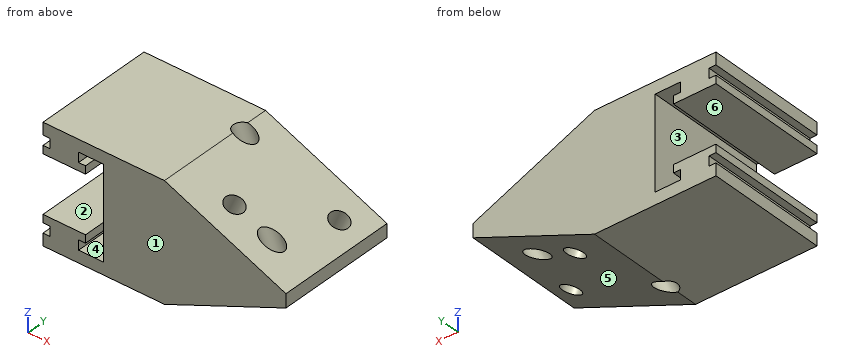
Autodesk Inventor part; units mm, degrees
ref_plane "YZ Plane" through (0, 0, 0) normal (1, 0, 0) x (0, 1, 0)
ref_plane "XZ Plane" through (0, 0, 0) normal (0, 1, 0) x (-1, 0, 0)
ref_plane "XY Plane" through (0, 0, 0) normal (0, 0, 1) x (1, 0, 0)
sketch "Sketch1" plane through (0, 0, 0) normal (0, 1, 0) x (-1, 0, 0)
  line L0 (0, 0) -> (-12.7, 0)
  line L1 (-12.7, 0) -> (-12.7, -2.54)
  line L2 (-12.7, -2.54) -> (0, -2.54)
  line L3 (0, -2.54) -> (0, 0)
  line L4 (0, -21.844) -> (-12.7, -21.844)
  line L5 (-12.7, -21.844) -> (-12.7, -24.384)
  line L6 (-12.7, -24.384) -> (0, -24.384)
  line L7 (0, -24.384) -> (0, -21.844)
  line L8 (-12.7, 0) -> (-25.4, 0)
  line L9 (-25.4, 0) -> (-25.4, -24.384)
  line L10 (-25.4, -24.384) -> (-12.7, -24.384)
  line L11 (-12.7, -24.384) -> (-12.7, 0)
  line L12 (-25.4, 0) -> (-50.8, -10.7817)
  line L13 (-25.4, 0) -> (2.1936, 0) construction
  line L14 (-25.4, -24.384) -> (-50.8, -13.6023)
  line L15 (-25.4, -24.384) -> (2.1936, -24.384) construction
  line L16 (-50.8, -10.7817) -> (-50.8, -13.6023)
  line L17 (-1.4478, -4.572) -> (-7.4422, -4.572)
  line L18 (-7.4422, -4.572) -> (-7.4422, -2.54)
  line L19 (-7.4422, -2.54) -> (-1.4478, -2.54)
  line L20 (-1.4478, -2.54) -> (-1.4478, -4.572)
  line L21 (-1.4478, -21.844) -> (-7.4422, -21.844)
  line L22 (-7.4422, -21.844) -> (-7.4422, -19.812)
  line L23 (-7.4422, -19.812) -> (-1.4478, -19.812)
  line L24 (-1.4478, -19.812) -> (-1.4478, -21.844)
  line L25 (0, -19.812) -> (-8.89, -19.812)
  line L26 (-8.89, -19.812) -> (-8.89, -18.161)
  line L27 (-8.89, -18.161) -> (0, -18.161)
  line L28 (0, -18.161) -> (0, -19.812)
  line L29 (0, -4.572) -> (-8.89, -4.572)
  line L30 (-8.89, -4.572) -> (-8.89, -6.223)
  line L31 (-8.89, -6.223) -> (0, -6.223)
  line L32 (0, -6.223) -> (0, -4.572)
  dimension "d2" = 12.7
  dimension "d3" = 2.54
  dimension "d4" = 12.7
  dimension "d5" = 2.54
  dimension "d6" = 24.384
  dimension "d7" = 12.7
  dimension "d8" = 24.384
  dimension "d9" = 157
  dimension "d10" = 157
  dimension "d11" = 25.4
  dimension "d12" = 25.4
  dimension "d15" = 5.9944
  dimension "d16" = 2.032
  dimension "d17" = 2.032
  dimension "d18" = 1.4478
  dimension "d19" = 5.9944
  dimension "d20" = 2.032
  dimension "d21" = 1.4478
  dimension "d22" = 8.89
  dimension "d23" = 1.651
  dimension "d24" = 8.89
  dimension "d25" = 1.651
extrude "Extrusion1" add sketch "Sketch1" along normal blind 25.4
sketch "Sketch2" plane through (25.4, 0, -24.384) normal (0.3907, 0, -0.9205) x (-0.9205, 0, -0.3907)
  circle A0 centre (-10.16, 19.05) radius 1.9685
  circle A1 centre (-22.5136, 6.35) radius 1.9685
  line L0 (-27.5936, 0) -> (0, 0)
  line L1 (-27.5936, 0) -> (-27.5936, 25.4)
  line L2 (0, 0) -> (0, 25.4)
  line L3 (-27.5936, 25.4) -> (0, 25.4)
  point P0 (13.8532, 0)
  dimension "d28" = 3.937
  dimension "d29" = 3.937
  dimension "d30" = 6.35
  dimension "d31" = 5.08
  dimension "d32" = 10.16
  dimension "d33" = 6.35
hole "Hole1" at (34.7523, 19.05, -20.4142) at (46.1238, 6.35, -15.5873) direction (-0.3907, 0, 0.9205) diameter 3.937 end through all
sketch "Sketch3" plane through (50.8, 0, -10.7817) normal (0.3907, 0, 0.9205) x (0.9205, 0, -0.3907)
  circle A0 centre (-5.08, 19.05) radius 1.9685
  circle A1 centre (-17.4336, 6.35) radius 1.9685
  line L0 (-27.5936, 25.4) -> (0, 25.4)
  line L1 (0, 0) -> (0, 25.4)
  line L2 (-27.5936, 0) -> (0, 0)
  line L3 (-27.5936, 0) -> (-27.5936, 17.1859)
  point P0 (-50.9744, 0)
  dimension "d41" = 3.937
  dimension "d42" = 3.937
  dimension "d43" = 6.35
  dimension "d44" = 5.08
  dimension "d45" = 6.35
  dimension "d46" = 10.16
hole "Hole2" at (46.1238, 19.05, -8.7967) at (34.7523, 6.35, -3.9698) direction (-0.3907, 0, -0.9205) diameter 3.937 end through all
ref_plane "Work Plane1" through (47.8226, 0, -17.7959) normal (0.3907, 0, 0.9205) x (0.9205, 0, -0.3907)
properties part number "XRailSplitter"
Check sheet for the modelled part. Datum: model origin and axes. Units: mm. Face numbers are marked on the shaded views. A direction names the side the tool comes from. Give positions to 0.01 mm unless a question says otherwise; leave off trailing zeros. Order: outer loops, then holes, each group sorted by start corner. A loop starts at its lowest first (then second) coordinate and runs counter-clockwise, first axis right, second up. Notation, with made-up numbers: M -23.75,79.25 L 33.25,79.25 A15 cw 33.25,95.25 Z; hole C -15,10.25 d8. An arc over 180 degrees is marked long. Answer in a Markdown table with one row per item. Add a question column.
Q1. Release check for a two-part mould opening along X. For the marked faces 3, 4, 5 and 6 record: released by +X, released by -X, zero draft, split by the parting line, or undercut.
Q2. Access from +Z, -Z, +X, -X, +Y, -Y to the whole of each face (thin tool, end or side, straight path). Record for the marked faces 1 and 2.
Q3. Thickness scan on L1, parallel to Z at x = 6, y = 22; L2, parallel to X at y = 18, z = -5.5; L3, parallel to Y at x = 28, z = -2.5. Record the ranges inside material, lowest first.
Q4. Sectioned sample at A-A, the plane y = 23.75. Record the boundary of the cut face in (x, z).
Q5. Gauge pin test, flat ends, axial feed: pin 1 Ø10 at (y, z) = (3.5, -20.5) entering from +X; pin 2 Ø0.5 at (y, z) = (13.5, -5) entering from +X; pin 3 Ø5 at (x, y) = (31, 22) entering from +Z. Record the tip position at first contact, or that the pin passes through.
Q6. Sectioned sample at B-B, the plane y = 20.25. Count the separate pieces of the cut face and the enclosed holes in it, and give its area (3 significant figures).
Verdict:
| question | item | result |
|---|---|---|
| 1 | face 3 | undercut |
| 1 | face 4 | undercut |
| 1 | face 5 | released by +X |
| 1 | face 6 | zero draft |
| 2 | face 1 | +Z, -Z, +X, -X, -Y |
| 2 | face 2 | -X, +Y, -Y |
| 3 | L1 | -24.38 to -18.16, -6.22 to 0 |
| 3 | L2 | 0 to 8.89, 12.7 to 26.61, 30.23 to 38.36 |
| 3 | L3 | 0 to 17.24, 20.86 to 25.4 |
| 4 | outline | M 0,-24.38 L 25.4,-24.38 L 50.8,-13.6 L 50.8,-10.78 L 25.4,0 L 0,0 L 0,-2.54 L 1.45,-2.54 L 1.45,-4.57 L 0,-4.57 L 0,-6.22 L 8.89,-6.22 L 8.89,-4.57 L 7.44,-4.57 L 7.44,-2.54 L 12.7,-2.54 L 12.7,-21.84 L 7.44,-21.84 L 7.44,-19.81 L 8.89,-19.81 L 8.89,-18.16 L 0,-18.16 L 0,-19.81 L 1.45,-19.81 L 1.45,-21.84 L 0,-21.84 Z |
| 5 | pin 1 | x = 46.33 |
| 5 | pin 2 | x = 37.77 |
| 5 | pin 3 | z = -1.32 |
| 6 | separate pieces | 3 |
| 6 | enclosed holes | 0 |
| 6 | area | 678 mm² |
